Design review of the part built by this model. Coordinates are the model's own, in mm. A direction names the side the tool comes from. Give positions to 0.01 mm unless a question says otherwise; leave off trailing zeros. Order: outer loops, then holes, each group sorted by start corner. A loop starts at its lowest first (then second) coordinate and runs counter-clockwise, first axis right, second up. Notation, with made-up numbers: M 79,-25 L 88,-25 A21 ccw 88,6 Z; hole C 47,29.5 d10. An arc over 180 degrees is marked long. Put each result on its own line as item: value. Start each with the question number.
from build123d import *

# Parameters (mm, degrees)
F3_D     = 7
F4_D     = 5
F5_D     = 7
F6_D     = 4
F7_SIZE  = 1
F8_SIZE  = 0.5
F9_SIZE  = 0.5
F10_SIZE = 0.5
F11_SIZE = 0.5


with BuildPart() as f1:
    # F0 (on Front) → F1 (revolve)
    with BuildSketch(Plane.XZ):
        Polygon((-55, 3), (-55, 0), (-40.5, 0), (-40.5, 6), (-23.51, 6), (-23.51, 9.8), (-25.25, 9.8), (-25.25, 11.65), (-23.51, 11.65), (-23.51, 30.65), (-19.37856, 30.65), (-19.37856, 32.65), (-26.81, 32.65), (-26.81, 12.921854), (-28.388953, 12.921854), (-28.388953, 10), (-43, 10), (-43, 3), align=None)
    revolve(axis=Axis((0, 0, 31.65), (0, 0, 1)))

    # F3 (through all)
    with Locations(Plane(origin=(0, 0, 0), x_dir=(1, 0, 0), z_dir=(0, 0, -1))):
        with Locations((-35.5, -35.5), (35.5, -35.5), (35.5, 35.5), (-35.5, 35.5)):
            Hole(F3_D / 2)

    # F4 (through all)
    with Locations(Plane(origin=(0, 0, 0), x_dir=(1, 0, 0), z_dir=(0, 0, -1))):
        with Locations((-18.353477, -44.309214), (18.353477, -44.309214), (44.309214, -18.353477), (44.309214, 18.353477), (18.353477, 44.309214), (-18.353477, 44.309214), (-44.309214, 18.353477), (-44.309214, -18.353477)):
            Hole(F4_D / 2)

    # F5 (through all)
    with Locations(Plane(origin=(0, 0, 0), x_dir=(1, 0, 0), z_dir=(0, 0, -1))):
        with Locations((0, -50.20458), (-50.20458, 0), (50.20458, 0), (0, 50.20458)):
            Hole(F5_D / 2)

    # F6 (through all)
    with Locations(Plane(origin=(0, 0, 0), x_dir=(1, 0, 0), z_dir=(0, 0, -1))):
        with Locations((-23.927569, 23.927569), (-8.758098, 32.685667), (8.758098, 32.685667), (23.927569, 23.927569), (32.685667, 8.758098), (32.685667, -8.758098), (23.927569, -23.927569), (8.758098, -32.685667), (-8.758098, -32.685667), (-23.927569, -23.927569), (-32.685667, -8.758098), (-32.685667, 8.758098)):
            Hole(F6_D / 2)

    # F7
    f7_edges = [f1.edges().sort_by_distance(p)[0] for p in [
        (23.51, 0, 6),
    ]]
    chamfer(f7_edges, length=F7_SIZE)

    # F8
    f8_edges = [f1.edges().sort_by_distance(p)[0] for p in [
        (55, 0, 3),
        (43, 0, 10),
        (28.388953, 0, 12.921854),
        (26.81, 0, 32.65),
    ]]
    chamfer(f8_edges, length=F8_SIZE)

    # F9
    f9_edges = [f1.edges().sort_by_distance(p)[0] for p in [
        (40.5, 0, 0),
    ]]
    chamfer(f9_edges, length=F9_SIZE)

    # F10
    f10_edges = [f1.edges().sort_by_distance(p)[0] for p in [
        (55, 0, 0),
    ]]
    chamfer(f10_edges, length=F10_SIZE)

    # F11
    f11_edges = [f1.edges().sort_by_distance(p)[0] for p in [
        (19.37856, 0, 32.65),
    ]]
    chamfer(f11_edges, length=F11_SIZE)


solid = f1.part
1. The part is to be moulded in two halves that separate along Y. For faces 1 (the cylindrical face through (46.866, -1.051, 1.521)), 2 (the cylindrical face through (6.154, 27.714, 11.194)), 3 (the cylindrical face through (-21.93, 23.84, 8.03)), 4 (the flat face through (40.1, -16.4, 3)), say which applies: +Y half, -Y half, draft (parallel to the pull), parting line (faces both ways), or undercut.
2. To check wall thickness, follow probe 1 along X at (y, z) = (35.5, 1.5); probe 2 along Y at (x, z) = (-0.5, 2); probe 3 along X at (y, z) = (0, 31.75). State the ranges of each line that lie inside material, in increasing order.
3. Consider section A-A on x = 0. Give the number of separate pieces and of enclosed holes in the cut face, then the cut area to 3 significant figures.
4. Consider section C-C on z = 29. Give the boundary of the cut face in (x, y), then the cut area to 3 significant figures.
5. Insertion check: pin 1 (6.5 mm diameter, centred on x = -35.5, y = 35.5, fed in from +Z); pin 2 (1 mm diameter, centred on x = -1.5, z = 27, fed in from -Y); pin 3 (3 mm diameter, centred on x = 24.5, z = 24, fed in from +Y); pin 4 (11 mm diameter, centred on x = -50.2, y = 0, fed in from +Z). Each pin has a flat end and moves straight along its axis. Give the tip position at first contact, or say it passes through.
6. Machinability: for faces 5 (the cylindrical face through (-41.81, 18.24, 1.52)), 6 (the cylindrical face through (5.598, -42.634, 6.204)), 7 (the cylindrical face through (-22.424, -7.062, 21.283)), which of the approach directions +Z, -Z, +X, -X, +Y, -Y give a long, thin tool a straight path to every point of the face, cutting with its end or side? Answer none if there is none.
Returned:
1. face 1: undercut
1. face 2: parting line
1. face 3: undercut
1. face 4: draft
2. probe 1: x = -42.01 to -39, -32 to -19.49, 19.49 to 32, 39 to 42.01
2. probe 2: y = -55 to -53.67, -46.74 to -40.5, 40.5 to 46.74, 53.67 to 55
2. probe 3: x = -26.81 to -19.38, 19.38 to 26.81
3. separate pieces: 4
3. enclosed holes: 0
3. area: 382 mm2
4. outline: C 0,0 d53.62; hole C 0,0 d47.02
4. area: 522 mm2
5. pin 1: passes through
5. pin 2: stops at y = -26.79
5. pin 3: stops at y = 13.78
5. pin 4: stops at z = 3
6. face 5: +Z, -Z
6. face 6: +Z
6. face 7: -Z
